Verification items for the finished model (mm, model axes). A direction names the side the tool comes from. Coordinates: 2 decimals unless noted, no trailing zeros. Order: outer loops, then holes, each group sorted by start corner. A loop starts at its lowest first (then second) coordinate and runs counter-clockwise, first axis right, second up. Notation, with made-up numbers: M -14.5,-13 L 6.5,-13 A23 ccw 6.5,4 Z; hole C 37.25,22 d2. An arc over 180 degrees is marked long. Answer as a JSON object with one key per item and string values. Group by question number.
(1) Mould release check, pull along Z, two halves, no side actions. Record for faces 4 (the face through (-7, -12, 34.5)), 5 (the face through (8.699, -10.715, 5.07)), 6 (the face through (0, -12, 0)): released by +Z, released by -Z, zero draft, split by the parting line, or undercut.
(2) Cross-section at D-D (z = 9). Enter the section's corners in (x, y), plus the area to 3 significant figures.
(3) Cross-section at B-B (z = 5). Count the separate pieces of the cut face and the enclosed holes in it, plus the area to 3 significant figures.
(4) Cross-section at A-A (x = -16). Enter the section's corners in (y, z), plus the area to 3 significant figures.
(5) Access from +Z, -Z, +X, -X, +Y, -Y to the whole of each face (thin tool, end or side, straight path). Record for faces 1 (the face through (-9, -5, 5)), 2 (the face through (4, -12, 23)), 3 (the face through (-4, -12, 23)).
(6) Gauge pin test, flat ends, axial feed: pin 1 Ø0.6 at (x, y) = (7.5, -12) entering from -Z; pin 2 Ø0.6 at (y, z) = (-11.5, 36.5) entering from -X; pin 3 Ø5.5 at (x, z) = (2, 18) entering from +Y; pin 4 Ø7 at (y, z) = (-5, 2.5) entering from -X. Record the tip position at first contact, or that the pin passes through.
(7) Cross-section at C-C (y = -4). Enter the section's corners in (x, z).
(8) Material ranges on line 1 (Z direction, x = -16, y = -0.8); line 2 (Y direction, x = 1, z = 7); line 3 (X direction, y = -2.75, z = 5.5), recorded low to high.
from build123d import *

# Parameters (mm, degrees)
PAD_DEPTH    = 10
SKETCH001_W  = 8
SKETCH001_H  = 2
PAD001_DEPTH = 30
SKETCH002_R  = 3
PAD002_DEPTH = 4
PAD002_TAPER = 6
SKETCH004_W  = 2
SKETCH004_H  = 5.5
PAD003_DEPTH = 5
SKETCH005_R  = 1.5
HOLE_DEPTH   = 2.001
FILLET_R     = 1
FILLET001_R  = 3
CHAMFER_SIZE = 2
FILLET002_R  = 1


with BuildPart() as part:
    # Sketch → Pad (new body)
    with BuildSketch(Plane.XY):
        Polygon((-21, 0), (-9, 0), (-9, -11), (0, -11), (0, -13), (-11, -13), (-11, -2), (-21, -2), align=None)
    pad = extrude(amount=PAD_DEPTH)

    # Mirrored: Pad across Sketch V_Axis
    add(pad.mirror(Plane(origin=(0, 0, 0), x_dir=(0, 0, 1), z_dir=(1, 0, 0))))

    # Sketch001 (on Face11 of Mirrored) → Pad001 (join)
    with BuildSketch(Plane.XY.offset(10)):
        with Locations((0, -12)):
            Rectangle(SKETCH001_W, SKETCH001_H)
    extrude(amount=PAD001_DEPTH)

    # Sketch002 (on Face13 of Pad001) → Pad002 (join)
    with BuildSketch(Plane(origin=(0, -11, 0), x_dir=(-1, 0, 0), z_dir=(0, 1, 0))):
        with Locations((0, 36)):
            Circle(SKETCH002_R)
    extrude(amount=PAD002_DEPTH, taper=PAD002_TAPER)

    # Sketch004 (on Face11 of Pad002) → Pad003 (join)
    with BuildSketch(Plane(origin=(-4, 0, 0), x_dir=(0, -1, 0), z_dir=(-1, 0, 0))):
        with Locations((12, 37.25)):
            Rectangle(SKETCH004_W, SKETCH004_H)
    pad003 = extrude(amount=PAD003_DEPTH)

    # Mirrored001: Pad003 across YZ
    add(pad003.mirror(Plane.YZ))

    # Sketch005 (on Face6 of Mirrored001) → Hole (cut, through all)
    with BuildSketch(Plane.XZ.offset(2)):
        with Locations((-16, 5)):
            Circle(SKETCH005_R)
        with Locations((16, 5)):
            Circle(SKETCH005_R)
    extrude(amount=-HOLE_DEPTH, mode=Mode.SUBTRACT)

    # Fillet
    fillet_edges = [part.edges().sort_by_distance(p)[0] for p in [
        (-21, -2, 5),
        (-11, -2, 5),
        (-11, -13, 5),
        (11, -13, 5),
        (21, -2, 5),
        (11, -2, 5),
        (9, -11, 5),
        (9, 0, 5),
        (-9, 0, 5),
        (-9, -11, 5),
    ]]
    fillet(fillet_edges, radius=FILLET_R)

    # Fillet001
    fillet001_edges = [part.edges().sort_by_distance(p)[0] for p in [
        (-4, -12, 10),
        (4, -12, 10),
    ]]
    fillet(fillet001_edges, radius=FILLET001_R)

    # Chamfer
    chamfer_edges = [part.edges().sort_by_distance(p)[0] for p in [
        (4, -12, 34.5),
        (-4, -12, 34.5),
    ]]
    chamfer(chamfer_edges, length=CHAMFER_SIZE)

    # Fillet002
    fillet002_edges = [part.edges().sort_by_distance(p)[0] for p in [
        (-9, -12, 34.5),
        (-9, -12, 40),
        (9, -12, 34.5),
        (9, -12, 40),
    ]]
    fillet(fillet002_edges, radius=FILLET002_R)


solid = part.part
Taken from the geometry:
{
 "1": {"face 4": "undercut", "face 5": "zero draft", "face 6": "released by -Z"},
 "2": {"outline": "M -21,-1 A1 ccw -20,-2 L -12,-2 A1 cw -11,-3 L -11,-12 A1 ccw -10,-13 L 10,-13 A1 ccw 11,-12 L 11,-3 A1 cw 12,-2 L 20,-2 A1 ccw 21,-1 L 21,0 L 10,0 A1 ccw 9,-1 L 9,-10 A1 cw 8,-11 L -8,-11 A1 cw -9,-10 L -9,-1 A1 ccw -10,0 L -21,0 Z", "area": "128 mm²"},
 "3": {"separate pieces": "3", "enclosed holes": "0", "area": "116 mm²"},
 "4": {"outline": "M -2,0 L 0,0 L 0,3.5 L -2,3.5 Z; M -2,6.5 L 0,6.5 L 0,10 L -2,10 Z", "area": "14.0 mm²"},
 "5": {"face 1": "+Z, -Z, +Y", "face 2": "+X, +Y, -Y", "face 3": "-X, +Y, -Y"},
 "6": {"pin 1": "stops at z = 0", "pin 2": "stops at x = -9", "pin 3": "stops at y = -11", "pin 4": "stops at x = -20.87"},
 "7": {"outline": "M -11,0 L -9,0 L -9,10 L -11,10 Z; M 9,0 L 11,0 L 11,10 L 9,10 Z"},
 "8": {"line 1": "z = 0 to 3.5, 6.5 to 10", "line 2": "y = -13 to -11", "line 3": "x = -11.03 to -9, 9 to 11.03"}
}
